Autodesk Inventor part; units mm, degrees
ref_plane "YZ Plane" through (0, 0, 0) normal (1, 0, 0) x (0, 1, 0)
ref_plane "XZ Plane" through (0, 0, 0) normal (0, 1, 0) x (-1, 0, 0)
ref_plane "XY Plane" through (0, 0, 0) normal (0, 0, 1) x (1, 0, 0)
sketch "Sketch1" plane through (0, 0, 0) normal (0, 1, 0) x (-1, 0, 0)
  line L0 (13.5, 4) -> (13.5, 5)
  line L1 (13.5, 5) -> (17.5, 5)
  line L2 (17.5, 5) -> (17.5, 10)
  line L3 (17.5, 10) -> (0, 10)
  line L4 (0, 10) -> (0, 0)
  line L5 (13.5, 4) -> (12.5, 4)
  line L6 (12.5, 4) -> (12.5, 0)
  line L7 (12.5, 0) -> (0, 0)
  dimension "d1" = 27
  dimension "d2" = 35
  dimension "d3" = 1
  dimension "d4" = 5
  dimension "d28" = 25
  dimension "d29" = 4
revolve "Revolution1" add sketch "Sketch1" angle 360 about axis through (0, 0, 10) along (0, 0, -1)
sketch "Sketch2" plane through (0, 0, 10) normal (0, 0, 1) x (1, 0, 0)
  point P0 (0, 0)
  point P1 (0, 9.5)
  dimension "d6" = 9.5
hole "Hole1" at (0, 9.5, 10) direction (0, 0, -1) diameter 3.4 end through all counterbore diameter 6.5 counterbore depth 4
pattern_circular "Circular Pattern1" count 6 over 360 about axis through (0, 0, -10) along (0, 0, -1) of "Hole1"
sketch "Sketch3" plane through (0, 0, 10) normal (0, 0, 1) x (1, 0, 0)
  point P0 (0, 0)
  point P1 (14, 0)
  dimension "d17" = 14
hole "Hole2" at (14, 0, 10) direction (0, 0, -1) diameter 2.459 end through all
pattern_circular "Circular Pattern2" count 6 over 360 about axis through (0, 0, -10) along (0, 0, 1) of "Hole2"
equation "\"d28\" = bearing_61705_inner"
equation "\"bearing_61807_inner\" = 35"
equation "\"bearing_61807_outer\" = 47.1"
equation "\"bearing_61814_outer\" = 90.1"
equation "\"bearing_61705_outer\" = 32.1"
equation "\"bearing_61705_inner\" = 25"
equation "\"M3_adjustable\" = 3.2"
equation "\"bearing_606_outer\" = 17.1"
equation "\"gearbox_35_outer\" = 32.3"
properties part number "405-output disk"
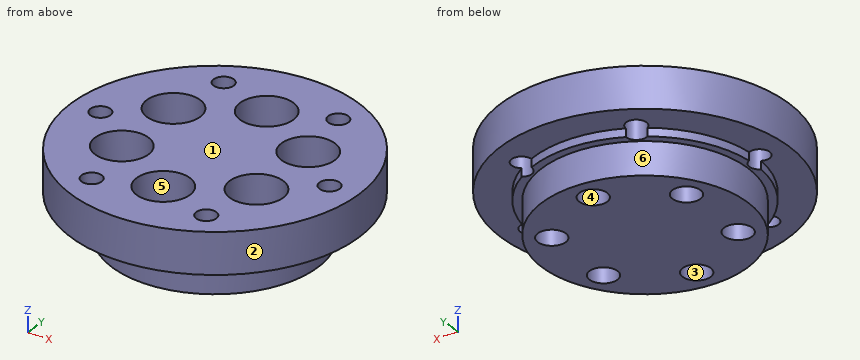
Geometry check sheet. Reference: the model listing, model coordinates, mm. Face numbers are marked on the shaded views. A direction names the side the tool comes from. Coordinates: 2 decimals unless noted, no trailing zeros. Loops run counter-clockwise (first coordinate to the right, second up) from the corner with the lowest first, then second, coordinate; pieces in that order, holes last.
Item 1: Sectioned sample at B-B, the plane y = 0. Record the boundary of the cut face in (x, z).
Item 2: Sectioned sample at C-C, the plane z = 3. Record the boundary of the cut face in (x, y) (3 decimals), then the cut area to 3 significant figures.
Item 3: Thickness scan on line 1 (X direction, y = 6, z = 1.75); line 2 (Y direction, x = -5.5, z = 7.5); line 3 (X direction, y = 7.5, z = 6.25). Record the ranges inside material, lowest first.
Item 4: Go/stop test with flat-tipped pins: pin 1 Ø1 at (y, z) = (-5, 3) entering from -X; pin 2 Ø1.5 at (y, z) = (-5.5, 4.5) entering from +X; pin 3 Ø6 at (y, z) = (-7.5, 6) entering from -X. Record where each tip stops, or that it passes through.
Item 5: Sectioned sample at A-A, the plane x = 0. Record the boundary of the cut face in (y, z).
Item 6: Access from +Z, -Z, +X, -X, +Y, -Y to the whole of each face (thin tool, end or side, straight path). Record for the marked faces 4, 5 and 6.
Item 7: Sectioned sample at D-D, the plane y = 9.5. Record the boundary of the cut face in (x, z).
Item 8: Release check for a two-part mould opening along Y. For the marked faces 1, 2 and 3 record: released by +Y, released by -Y, zero draft, split by the parting line, or undercut.
Check result:
1. outline: (-17.5, 5) - (-15.23, 5) - (-15.23, 10) - (-17.5, 10) - close; (-12.77, 4) - (-12.5, 4) - (-12.5, 0) - (12.5, 0) - (12.5, 4) - (12.77, 4) - (12.77, 10) - (-12.77, 10) - close; (15.23, 5) - (17.5, 5) - (17.5, 10) - (15.23, 10) - close
2. outline: circle Ø25 at (0, 0); hole circle Ø3.4 at (-8.227, -4.75); hole circle Ø3.4 at (-8.227, 4.75); hole circle Ø3.4 at (0, -9.5); hole circle Ø3.4 at (0, 9.5); hole circle Ø3.4 at (8.227, -4.75); hole circle Ø3.4 at (8.227, 4.75)
2. area: 436 mm2
3. line 1: x = -10.97 to -9.38, -7.08 to 7.08, 9.38 to 10.97
3. line 2: y = -16.61 to -6.52, -2.98 to 2.98, 6.52 to 16.61
3. line 3: x = -15.81 to -9.96, -6.5 to -2.56, 2.56 to 6.5, 9.96 to 15.81
4. pin 1: stops at x = -11.66
4. pin 2: stops at x = 16.79
4. pin 3: stops at x = -16.91
5. outline: (-17.5, 5) - (-13.5, 5) - (-13.5, 4) - (-12.5, 4) - (-12.5, 0) - (-11.2, 0) - (-11.2, 6) - (-12.75, 6) - (-12.75, 10) - (-17.5, 10) - close; (-7.8, 0) - (7.8, 0) - (7.8, 6) - (6.25, 6) - (6.25, 10) - (-6.25, 10) - (-6.25, 6) - (-7.8, 6) - close; (11.2, 0) - (12.5, 0) - (12.5, 4) - (13.5, 4) - (13.5, 5) - (17.5, 5) - (17.5, 10) - (12.75, 10) - (12.75, 6) - (11.2, 6) - close
6. face 4: +Z, -Z
6. face 5: +Z
6. face 6: -Z
7. outline: (-14.7, 5) - (-9.59, 5) - (-9.59, 4) - (-8.12, 4) - (-8.12, 0) - (-1.7, 0) - (-1.7, 6) - (-3.25, 6) - (-3.25, 10) - (-14.7, 10) - close; (1.7, 0) - (8.12, 0) - (8.12, 4) - (9.59, 4) - (9.59, 5) - (14.7, 5) - (14.7, 10) - (3.25, 10) - (3.25, 6) - (1.7, 6) - close
8. face 1: zero draft
8. face 2: split by the parting line
8. face 3: undercut
